Input: part model. Units: mm. Frame: model coordinates. A direction names the side the tool comes from. Coordinates: 2 decimals unless noted, no trailing zeros. Loops run counter-clockwise (first coordinate to the right, second up) from the corner with the lowest first, then second, coordinate; pieces in that order, holes last. Notation, with made-up numbers: (35, -31) - (79, -31) arc R21 cw to (79, 4) - close; hole circle Ø4 at (27.5, 10.25). An arc over 180 degrees is marked (long way). Use one line per item in the form item = value.
from build123d import *

# Parameters (mm, degrees)
SKETCH2_R           = 4
SKETCH2_R_2         = 1.925
BOSS_EXTRUDE1_DEPTH = 27
SKETCH3_R           = 4.05
CUT_EXTRUDE1_DEPTH  = 25
SKETCH5_W           = 9
SKETCH5_H           = 9
CUT_EXTRUDE2_DEPTH  = 25
SKETCH6_R           = 1.825
CUT_EXTRUDE3_DEPTH  = 5


with BuildPart() as part:
    # Sketch2 → Boss-Extrude1 (new body)
    # profile 1 of 2: a face of its own
    with BuildSketch(Plane(origin=(0, 0, 0), x_dir=(1, 0, 0), z_dir=(0, 1, 0))):
        Circle(SKETCH2_R)
        with Locations(Location((0, 0, 0), (0, 0, 270))):
            Circle(SKETCH2_R_2, mode=Mode.SUBTRACT)
    # profile 2 of 2: a face of its own
    with BuildSketch(Plane(origin=(0, 0, 0), x_dir=(1, 0, 0), z_dir=(0, 1, 0))):
        with BuildLine():
            ThreePointArc((4, 0), (0, -4), (-4, 0))
            Line((-4, 0), (-4, -20))
            Line((-4, -20), (4, -20))
            Line((4, -20), (4, 0))
        make_face()
    extrude(amount=BOSS_EXTRUDE1_DEPTH)

    # Sketch3 → Cut-Extrude1 (cut)
    with BuildSketch(Plane(origin=(4, 0, 0), x_dir=(0, 0, -1), z_dir=(1, 0, 0))):
        with Locations((-14, 21)):
            Circle(SKETCH3_R)
    extrude(amount=-CUT_EXTRUDE1_DEPTH, mode=Mode.SUBTRACT)

    # Sketch5 → Cut-Extrude2 (cut)
    with BuildSketch(Plane.ZY.offset(4)):
        with Locations((0.5, 13.5)):
            Rectangle(SKETCH5_W, SKETCH5_H)
    extrude(amount=-CUT_EXTRUDE2_DEPTH, mode=Mode.SUBTRACT)

    # Sketch6 → Cut-Extrude3 (cut)
    with BuildSketch(Plane(origin=(0, 0, 0), x_dir=(-1, 0, 0), z_dir=(0, -1, 0))):
        with Locations(Location((0, -15, 0), (0, 0, 90))):
            Circle(SKETCH6_R)
    extrude(amount=-CUT_EXTRUDE3_DEPTH, mode=Mode.SUBTRACT)


solid = part.part
Q1. Cut plane B-B, the plane y = 21. Return loops of the section in (x, z) (3 decimals), then the cut area to 3 significant figures.
Check values:
outline = (-4, 0) arc R4 ccw to (4, 0) - (4, 9.95) - (-4, 9.95) - close; (-4, 18.05) - (4, 18.05) - (4, 20) - (-4, 20) - close; hole circle Ø3.85 at (0, 0)
area = 109 mm²
Q2. Set-up query: faces 4 (the flat face through (-0.1, 18, 2.4)), 5 (the cylindrical face through (0.08, 2.465, 16.823)), 6 (the cylindrical face through (0.056, 18.536, 17.214)). Return all of +Z, -Z, +X, -X, +Y, -Y with unobstructed straight access to the full face (end or side cutting, diameter ignored); none if empty.
Check values:
face_4 = -Z, +X, -X
face_5 = -Y
face_6 = +X, -X
Q3. First-contact query: P1, Ø1.1, axis at x = -0.5, z = 15.5, coming from the -Y side; P2, Ø8, axis at y = 18, z = 13.5, coming from the -X side. Flat tips, straight axial feed; report the tip coordinate or a pass-through.
Check values:
P1 = 5
P2 = -4
Q4. Ray query, line 1 along Y through (x, z) = (-2, 14); line 2 along Y through (x, z) = (1, 14); line 3 along Z through (x, y) = (0, 23) (3 decimals). Return the intervals inside material, ascending. Write a range as [from, to].
Check values:
line_1 = [0, 16.95], [25.05, 27]
line_2 = [5, 16.95], [25.05, 27]
line_3 = [-4, -1.925], [1.925, 10.478], [17.522, 20]
Q5. Pull-direction query (Z, two-part tool) for faces 1 (the cylindrical face through (-1.17, 22.44, -1.53)), 2 (the flat face through (-0.1, 9, 2.4)), 3 (the cylindrical face through (0, 22, -4)); classes: pulls with the +Z half, pulls with the -Z half, needs draft (parallel to the pull), parting line crosses it, or undercut.
Check values:
face_1 = undercut
face_2 = needs draft
face_3 = pulls with the -Z half
Q6. Cut plane D-D, the plane x = -2.25. Return loops of the section in (y, z), then the cut area to 3 significant figures.
Check values:
outline = (0, -3.31) - (9, -3.31) - (9, 5) - (18, 5) - (18, -3.31) - (27, -3.31) - (27, 20) - (0, 20) - close; hole circle Ø8.1 at (21, 14)
area = 503 mm²
Q7. Cut plane C-C, the plane z = 10.25. Return loops of the section in (x, y).
Check values:
outline = (-4, 0) - (4, 0) - (4, 19.47) - (-4, 19.47) - close; (-4, 22.53) - (4, 22.53) - (4, 27) - (-4, 27) - close
Q8. Cut plane A-A, the plane x = 0. Return loops of the section in (y, z) (3 decimals), then the cut area to 3 significant figures.
Check values:
outline = (0, -4) - (9, -4) - (9, -1.925) - (0, -1.925) - close; (0, 1.925) - (9, 1.925) - (9, 5) - (18, 5) - (18, 1.925) - (27, 1.925) - (27, 20) - (0, 20) - (0, 16.825) - (5, 16.825) - (5, 13.175) - (0, 13.175) - close; (18, -4) - (27, -4) - (27, -1.925) - (18, -1.925) - close; hole circle Ø8.1 at (21, 14)
area = 428 mm²
